The model under review builds one solid part; all positions refer to its coordinate system, in mm. Face numbers are marked on the shaded views. A direction names the side the tool comes from. Coordinates: 2 decimals unless noted, no trailing zeros. Order: outer loops, then holes, each group sorted by start corner. A loop starts at its lowest first (then second) coordinate and runs counter-clockwise, first axis right, second up. Notation, with made-up numbers: (52.5, -2.75) - (109.5, -2.75) arc R5 cw to (109.5, 2.25) - close; hole circle Ø7 at (25.25, -21). An arc over 180 degrees is marked (long way). Answer in a Markdown table with one row per item.
```python
from build123d import *

# Parameters (mm, degrees)
SKETCH1_R           = 17
SKETCH1_R_2         = 6.35
BOSS_EXTRUDE1_DEPTH = 12
FILLET1_R           = 1
SKETCH2_R           = 14.179085796
SKETCH2_R_2         = 9.276544236
CUT_EXTRUDE1_DEPTH  = 1
SKETCH3_R           = 14.472019466
SKETCH3_R_2         = 9.262101897
CUT_EXTRUDE2_DEPTH  = 1


with BuildPart() as part:
    # Sketch1 → Boss-Extrude1 (new body)
    with BuildSketch(Plane(origin=(0, 0, 0), x_dir=(1, 0, 0), z_dir=(0, 1, 0))):
        Circle(SKETCH1_R)
        Circle(SKETCH1_R_2, mode=Mode.SUBTRACT)
    extrude(amount=BOSS_EXTRUDE1_DEPTH)

    # Fillet1
    fillet1_edges = [part.edges().sort_by_distance(p)[0] for p in [
        (-17, 0, 0),
        (-17, 12, 0),
        (-6.35, 0, 0),
        (-6.35, 12, 0),
    ]]
    fillet(fillet1_edges, radius=FILLET1_R)

    # Sketch2 → Cut-Extrude1 (cut)
    with BuildSketch(Plane(origin=(0, 12, 0), x_dir=(1, 0, 0), z_dir=(0, 1, 0))):
        Circle(SKETCH2_R)
        Circle(SKETCH2_R_2, mode=Mode.SUBTRACT)
    extrude(amount=-CUT_EXTRUDE1_DEPTH, mode=Mode.SUBTRACT)

    # Sketch3 → Cut-Extrude2 (cut)
    with BuildSketch(Plane.XZ):
        Circle(SKETCH3_R)
        Circle(SKETCH3_R_2, mode=Mode.SUBTRACT)
    extrude(amount=-CUT_EXTRUDE2_DEPTH, mode=Mode.SUBTRACT)


solid = part.part
```
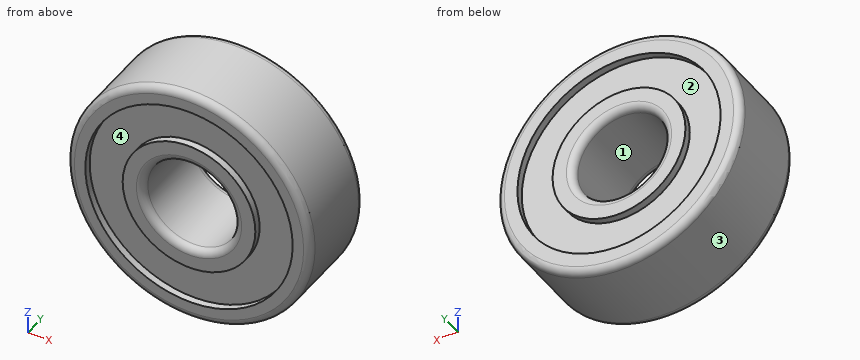
Item 1: We need section C-C, the plane y = 7.5. Write out the cut boundary in (x, z), then the cut area to 3 significant figures.
Check values:
| item | result |
|---|---|
| outline | circle Ø34 at (0, 0); hole circle Ø12.7 at (0, 0) |
| area | 781 mm^2 |
Item 2: Clearance check with flat-ended pins moving along their axes: pin 1 Ø1.5 at (y, z) = (6.5, 4) entering from +X; pin 2 Ø3 at (y, z) = (2, -8.5) entering from -X; pin 3 Ø2 at (x, y) = (11, 2.5) entering from -Z; pin 4 Ø10 at (x, z) = (0, 0) entering from -Y. State where each tip first meets the part, or that it passes through.
Check values:
| item | result |
|---|---|
| pin 1 | x = 16.69 |
| pin 2 | x = -15.49 |
| pin 3 | z = -13.75 |
| pin 4 | through |
Item 3: To check wall thickness, follow line 1 (Z direction, x = 0, y = 5); line 2 (Z direction, x = 0, y = 11.35). State the ranges of each line that lie inside material, in increasing order. Write a range as from..to.
Check values:
| item | result |
|---|---|
| line 1 | -17..-6.35, 6.35..17 |
| line 2 | -16.94..-14.18, -9.28..-6.41, 6.41..9.28, 14.18..16.94 |
Item 4: Tool access review of the marked faces 1 and 2: name each direction out of +Z, -Z, +X, -X, +Y, -Y from which nothing blocks a thin tool from reaching the whole face with its end or side.
Check values:
| item | result |
|---|---|
| face 1 | +Y, -Y |
| face 2 | +Y |
Item 5: Mouldability with a two-part tool opening along Z and no side actions: class the marked faces 3 and 4 as +Z half, -Z half, draft (parallel to the pull), parting line (faces both ways), or undercut.
Check values:
| item | result |
|---|---|
| face 3 | parting line |
| face 4 | undercut |
